```python
from build123d import *

# Parameters (mm, degrees)
CROQUIS1_R              = 1.5
SALIENTE_EXTRUIR1_DEPTH = 4
CROQUIS2_R              = 11.5
SALIENTE_EXTRUIR2_DEPTH = 7


with BuildPart() as part:
    # Croquis1 → Saliente-Extruir1 (new body)
    with BuildSketch(Plane(origin=(0, 0, 0), x_dir=(1, 0, 0), z_dir=(0, 1, 0))):
        with BuildLine():
            Line((16.5, 2), (6.9, 9.2))
            ThreePointArc((6.9, 9.2), (0, 11.5), (-6.9, 9.2))
            Line((-6.9, 9.2), (-16.5, 2))
            ThreePointArc((-16.5, 2), (-17.5, 0), (-16.5, -2))
            Line((-16.5, -2), (-6.9, -9.2))
            ThreePointArc((-6.9, -9.2), (0, -11.5), (6.9, -9.2))
            Line((6.9, -9.2), (16.5, -2))
            ThreePointArc((16.5, -2), (17.5, 0), (16.5, 2))
        make_face()
        with Locations(Location((-15, 0, 0), (0, 0, 270))):
            Circle(CROQUIS1_R, mode=Mode.SUBTRACT)
        with Locations(Location((15, 0, 0), (0, 0, 270))):
            Circle(CROQUIS1_R, mode=Mode.SUBTRACT)
    extrude(amount=SALIENTE_EXTRUIR1_DEPTH)

    # Croquis2 → Saliente-Extruir2 (add)
    with BuildSketch(Plane(origin=(0, 4, 0), x_dir=(1, 0, 0), z_dir=(0, 1, 0))):
        with Locations(Location((0, 0, 0), (0, 0, 53.130102354))):
            Circle(CROQUIS2_R)
    extrude(amount=SALIENTE_EXTRUIR2_DEPTH)


solid = part.part
```
Geometry: final body of the model. Coordinates: model frame, mm. Round coordinates to 2 decimals unless told otherwise and drop trailing zeros. Order: outer loops, then holes, each group sorted by start corner. A loop starts at its lowest first (then second) coordinate and runs counter-clockwise, first axis right, second up. Notation, with made-up numbers: (59.5, 87) - (101.5, 87) arc R26 cw to (101.5, 119) - close; hole circle Ø9 at (-16.75, -3). An arc over 180 degrees is marked (long way). Use CSV: the item, a comma, the result in double quotes. Start each with the question number.
Q1. Section query D-D (z = 5.25). Return loops of the section in (x, y).
Q2. Section query A-A (y = 1.75). Return loops of the section in (x, z).
Q3. Section query B-B (z = 0). Return loops of the section in (x, y).
Q4. Mould query, pull axis Z, two halves, no side actions, for faces 1 (the face through (11.77, 1.97, -5.55)), 2 (the face through (16.265, 1.972, 0.806)), 3 (the face through (-14.55, 1.97, 1.43)), 4 (the face through (-13, 4, -1)). Classes: +Z half, -Z half, draft (parallel to the pull), parting line (faces both ways), or undercut.
Q5. Section query C-C (x = -15). Return loops of the section in (y, z) (3 decimals).
Q6. Material intervals for line 1 along Y through (x, z) = (-13, -3); line 2 along X through (y, z) = (4.5, -3.75); line 3 along X through (y, z) = (10, 4.25), sorted ascending. Write a range as from..to.
Q7. First-contact query: pin 1 (2.5 mm diameter, centred on x = 15, z = 0, fed in from -Y); pin 2 (4 mm diameter, centred on y = 8.5, z = -8, fed in from -X); pin 3 (2 mm diameter, centred on y = 1.5, z = 8, fed in from +X). Flat tips, straight axial feed; report the tip coordinate or a pass-through.
Result set:
1,outline,"(-12.17, 0) - (12.17, 0) - (12.17, 4) - (10.23, 4) - (10.23, 11) - (-10.23, 11) - (-10.23, 4) - (-12.17, 4) - close"
2,outline,"(-16.5, -2) - (-6.9, -9.2) arc R11.5 ccw to (6.9, -9.2) - (16.5, -2) arc R2.5 ccw to (16.5, 2) - (6.9, 9.2) arc R11.5 ccw to (-6.9, 9.2) - (-16.5, 2) arc R2.5 ccw to start; hole circle Ø3 at (-15, 0); hole circle Ø3 at (15, 0)"
3,outline,"(-17.5, 0) - (-16.5, 0) - (-16.5, 4) - (-17.5, 4) - close; (-13.5, 0) - (13.5, 0) - (13.5, 4) - (11.5, 4) - (11.5, 11) - (-11.5, 11) - (-11.5, 4) - (-13.5, 4) - close; (16.5, 0) - (17.5, 0) - (17.5, 4) - (16.5, 4) - close"
4,face 1,"-Z half"
4,face 2,"undercut"
4,face 3,"undercut"
4,face 4,"draft"
5,outline,"(0, -3.125) - (4, -3.125) - (4, -1.5) - (0, -1.5) - close; (0, 1.5) - (4, 1.5) - (4, 3.125) - (0, 3.125) - close"
6,line 1,"y = 0..4"
6,line 2,"x = -10.87..10.87"
6,line 3,"x = -10.69..10.69"
7,pin 1,"passes through"
7,pin 2,"stops at x = -9.81"
7,pin 3,"stops at x = 9.83"
